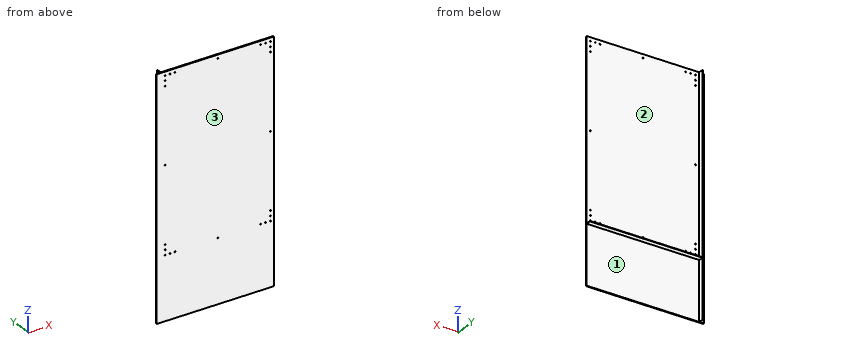
from build123d import *

# Parameters (mm, degrees)
SKETCH1_W                  = 609.6
SKETCH1_H                  = 1219.2
BOSS_EXTRUDE1_DEPTH        = 5.5
SKETCH2_W                  = 584.2
SKETCH2_H                  = 2.54
EXTRUDE_THIN1_DEPTH        = 25.4
SKETCH2_3_W                = 2.54
SKETCH2_3_H                = 1219.2
EXTRUDE_THIN2_DEPTH        = 25.4
F_5_3_5_3_DIAMETER_HOLE1_D = 5.3


with BuildPart() as part:
    # Sketch1 → Boss-Extrude1 (new body)
    with BuildSketch(Plane(origin=(0, 0, 0), x_dir=(1, 0, 0), z_dir=(0, 1, 0))):
        Rectangle(SKETCH1_W, SKETCH1_H)
    extrude(amount=BOSS_EXTRUDE1_DEPTH)

    # Sketch2 → Extrude-Thin1 (add)
    with BuildSketch(Plane(origin=(0, 5.5, 0), x_dir=(1, 0, 0), z_dir=(0, 1, 0))):
        with Locations((12.7, 306.07)):
            Rectangle(SKETCH2_W, SKETCH2_H)
    extrude(amount=EXTRUDE_THIN1_DEPTH)

    # Sketch2_3 → Extrude-Thin2 (add)
    with BuildSketch(Plane(origin=(0, 5.5, 0), x_dir=(1, 0, 0), z_dir=(0, 1, 0))):
        with Locations((-280.67, 0)):
            Rectangle(SKETCH2_3_W, SKETCH2_3_H)
    extrude(amount=EXTRUDE_THIN2_DEPTH)

    # 5.3 _5.3_ Diameter Hole1 (through all)
    with Locations(Plane(origin=(0, 5.5, 0), x_dir=(1, 0, 0), z_dir=(0, 1, 0))):
        with Locations((-260.35, 285.75), (-234.95, 285.75), (-209.55, 285.75), (-260.35, 260.35), (-260.35, 234.95), (12.7, 285.75), (234.95, 285.75), (260.35, 285.75), (285.75, 285.75), (285.75, 260.35), (285.75, 234.95), (-260.35, -152.4), (285.75, -152.4), (-260.35, -539.75), (-260.35, -565.15), (-260.35, -590.55), (-234.95, -590.55), (-209.55, -590.55), (12.7, -590.55), (234.95, -590.55), (260.35, -590.55), (285.75, -590.55), (285.75, -565.15), (285.75, -539.75)):
            Hole(F_5_3_5_3_DIAMETER_HOLE1_D / 2)


solid = part.part
Design review of the part built by this model. Coordinates are the model's own, in mm. Face numbers are marked on the shaded views. A direction names the side the tool comes from. Round coordinates to 2 decimals unless told otherwise and drop trailing zeros. Loops run counter-clockwise (first coordinate to the right, second up) from the corner with the lowest first, then second, coordinate; pieces in that order, holes last. Notation, with made-up numbers: (21.25, 41) - (33.25, 41) arc R17 cw to (33.25, 59) - close; hole circle Ø5 at (68.25, 74). An arc over 180 degrees is marked (long way). One line per question, with ' | ' between items.
1. Clearance check with flat-ended pins moving along their axes: P1, Ø12.5, axis at x = 80.5, y = 14.5, coming from the +Z side; P2, Ø3, axis at y = 27, z = 261.5, coming from the +X side; P3, Ø3, axis at x = 127, y = 15, coming from the -Z side. State where each tip first meets the part, or that it passes through.
Results are:
P1: stops at z = -304.8 | P2: stops at x = -279.4 | P3: stops at z = -307.34
2. For the marked faces 1, 2 and 3, list the 3-axis set-ups (+Z, -Z, +X, -X, +Y, -Y) from which the entire face can be reached by the end or side of a thin tool; tool diameter is ignored.
Results are:
face 1: -Z, +X, +Y | face 2: +Z, +X, +Y | face 3: +Z, -Z, +X, -X, -Y
3. We need section B-B, the plane z = -47. State the section outline as (x, y) points, and give its area (3 significant figures).
Results are:
outline: (-304.8, 0) - (304.8, 0) - (304.8, 5.5) - (-279.4, 5.5) - (-279.4, 30.9) - (-281.94, 30.9) - (-281.94, 5.5) - (-304.8, 5.5) - close | area: 3,420 mm²
4. We need section A-A, the plane x = -32.5. State the section outline as (y, z) points, and give its area (3 significant figures).
Results are:
outline: (0, -609.6) - (5.5, -609.6) - (5.5, -307.34) - (30.9, -307.34) - (30.9, -304.8) - (5.5, -304.8) - (5.5, 609.6) - (0, 609.6) - close | area: 6,770 mm²
5. For L1, parallel to X at y = 1.6, z = 539.75; L2, parallel to Z at x = -234.95, y = 2.35; L3, parallel to Z at x = 12, y = 11.5, list the stretches that pass through material, from the lowest coordinate up. Write a range as [from, to].
Results are:
L1: x = [-304.8, -263], [-257.7, 283.1], [288.4, 304.8] | L2: z = [-609.6, -288.4], [-283.1, 587.9], [593.2, 609.6] | L3: z = [-307.34, -304.8]
